Answer from the drawing. Dimensions are ordinates in mm from the lowest x, y and z of the part. Round coordinates to 2 decimals unless told otherwise and drop trailing zeros. Loops run counter-clockwise (first coordinate to the right, second up) from the corner with the lowest first, then second, coordinate; pieces in that order, holes last. Notation, with made-up numbers: (52, 39) - (69, 39) arc R9 ccw to (69, 46) - close; hole circle Ø5 at (18.25, -36.5). An arc over 180 degrees is marked (long way). Return JSON: item names as keys, results as strings.
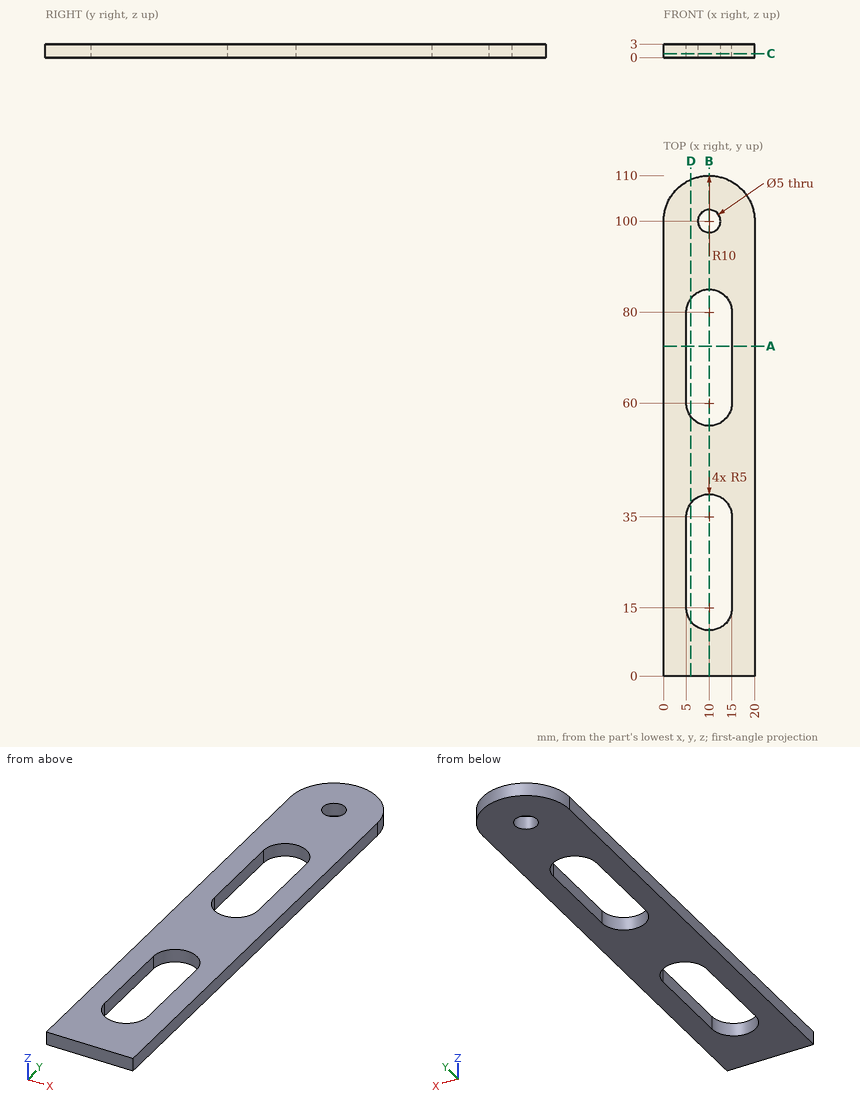
1) Section D-D (x = 6) is taken. Give the vertices of the cut face in (y, z), and give its area (3 significant figures).
Verdict:
{"outline": "(0, 0) - (12, 0) - (12, 3) - (0, 3) - close; (38, 0) - (57, 0) - (57, 3) - (38, 3) - close; (83, 0) - (109.17, 0) - (109.17, 3) - (83, 3) - close", "area": "171 mm2"}
2) A flat-ended cylindrical pin translates along its axis: pin 1 (3 mm diameter, centred on x = 10, y = 100, fed in from +Z). Find the tip coordinate at first contact, or state that the pin passes through.
Verdict:
{"pin 1": "passes through"}
3) Section B-B (x = 10) is taken. Give the vertices of the cut face in (y, z).
Verdict:
{"outline": "(0, 0) - (10, 0) - (10, 3) - (0, 3) - close; (40, 0) - (55, 0) - (55, 3) - (40, 3) - close; (85, 0) - (97.5, 0) - (97.5, 3) - (85, 3) - close; (102.5, 0) - (110, 0) - (110, 3) - (102.5, 3) - close"}
4) Find the intervals of material crossed by L1, parallel to Y at x = 10, z = 0.65; L2, parallel to Y at x = 14.5, z = 1.4; L3, parallel to Y at x = 9, z = 0.9, in increasing order.
Verdict:
{"L1": "y = 0 to 10, 40 to 55, 85 to 97.5, 102.5 to 110", "L2": "y = 0 to 12.82, 37.18 to 57.82, 82.18 to 108.93", "L3": "y = 0 to 10.1, 39.9 to 55.1, 84.9 to 97.71, 102.29 to 109.95"}
5) Section C-C (z = 0.9) is taken. Give the vertices of the cut face in (x, y).
Verdict:
{"outline": "(0, 0) - (20, 0) - (20, 100) arc R10 ccw to (0, 100) - close; hole (5, 15) arc R5 ccw to (15, 15) - (15, 35) arc R5 ccw to (5, 35) - close; hole (5, 60) arc R5 ccw to (15, 60) - (15, 80) arc R5 ccw to (5, 80) - close; hole circle Ø5 at (10, 100)"}
6) Section A-A (y = 72.5) is taken. Give the vertices of the cut face in (x, z).
Verdict:
{"outline": "(0, 0) - (5, 0) - (5, 3) - (0, 3) - close; (15, 0) - (20, 0) - (20, 3) - (15, 3) - close"}
